```python
from build123d import *

# Parameters (mm, degrees)
F0_W     = 100
F0_H     = 100
F1_DEPTH = 100
F2_R     = 5
F3_DEPTH = 10
F4_R     = 5
F5_DEPTH = 10
F7_D     = 10


with BuildPart() as f1:
    # F0 (on Front) → F1 (new body)
    with BuildSketch(Plane.XZ):
        Rectangle(F0_W, F0_H)
    extrude(amount=F1_DEPTH)

    # F2 (on face) → F3 (join)
    with BuildSketch(Plane.XZ.offset(100)):
        Circle(F2_R)
    extrude(amount=F3_DEPTH)

    # F4 (on face) → F5 (join)
    with BuildSketch(Plane(origin=(0, 0, -50), x_dir=(1, 0, 0), z_dir=(0, 0, -1))):
        with Locations((0.200286, 29.510024)):
            Circle(F4_R)
    extrude(amount=F5_DEPTH)

    # F7 (through all)
    with Locations(Plane.YZ.offset(50)):
        with Locations((-50.594613, 0)):
            Hole(F7_D / 2)


solid = f1.part
```
Geometry check sheet. Reference: the model listing, model coordinates, mm. A direction names the side the tool comes from. Round coordinates to 2 decimals unless told otherwise and drop trailing zeros. Loops run counter-clockwise (first coordinate to the right, second up) from the corner with the lowest first, then second, coordinate; pieces in that order, holes last. Notation, with made-up numbers: (1.5, 13) -> (21.5, 13) arc R19 ccw to (21.5, 39) -> close; hole circle Ø1 at (-23.75, -3.75). An arc over 180 degrees is marked (long way). Use a Markdown table: item, result.
(1) Sectioned sample at D-D (x = 0). Enter the section's corners in (y, z), then the cut area to 3 significant figures.
Calculated:
| item | result |
|---|---|
| outline | (-110, -5) -> (-100, -5) -> (-100, -50) -> (-34.51, -50) -> (-34.51, -60) -> (-24.51, -60) -> (-24.51, -50) -> (0, -50) -> (0, 50) -> (-100, 50) -> (-100, 5) -> (-110, 5) -> close; hole circle Ø10 at (-50.59, 0) |
| area | 10,100 mm² |
(2) Sectioned sample at A-A (z = 0). Enter the section's corners in (x, y).
Calculated:
| item | result |
|---|---|
| outline | (-50, -100) -> (-5, -100) -> (-5, -110) -> (5, -110) -> (5, -100) -> (50, -100) -> (50, -55.59) -> (-50, -55.59) -> close; (-50, -45.59) -> (50, -45.59) -> (50, 0) -> (-50, 0) -> close |
(3) Scan lines: probe 1 along Z at (x, y) = (28.5, -59); probe 2 along Y at (x, z) = (10, -48.5). Record each from-to range of solid material in increasing order.
Calculated:
| item | result |
|---|---|
| probe 1 | -50 to 50 |
| probe 2 | -100 to 0 |
(4) Sectioned sample at C-C (y = -96). Enter the section's corners in (x, z), then the cut area to 3 significant figures.
Calculated:
| item | result |
|---|---|
| outline | (-50, -50) -> (50, -50) -> (50, 50) -> (-50, 50) -> close |
| area | 10,000 mm² |
(5) Go/stop test with flat-tipped pins: P1, Ø4, axis at x = 34.5, y = -97, coming from the -Z side; P2, Ø1.5, axis at x = 3, z = -11.5, coming from the -Y side; P3, Ø13, axis at y = -50.59, z = 0, coming from the +X side. Record where each tip stops, or that it passes through.
Calculated:
| item | result |
|---|---|
| P1 | z = -50 |
| P2 | y = -100 |
| P3 | x = 50 |
(6) Sectioned sample at B-B (x = -21.5). Enter the section's corners in (y, z), then the cut area to 3 significant figures.
Calculated:
| item | result |
|---|---|
| outline | (-100, -50) -> (0, -50) -> (0, 50) -> (-100, 50) -> close; hole circle Ø10 at (-50.59, 0) |
| area | 9,920 mm² |
(7) Mould release check, pull along Z, two halves, no side actions. Record for faces 1 (the cylindrical face through (-0.88, -24.63, -54.93)), 2 (the cylindrical face through (-0.7, -55.364, 1.502)), 3 (the flat face through (0, -30, -60)): released by +Z, released by -Z, zero draft, split by the parting line, or undercut.
Calculated:
| item | result |
|---|---|
| face 1 | zero draft |
| face 2 | undercut |
| face 3 | released by -Z |
(8) Set-up check for faces 4 (the cylindrical face through (-1.08, -104.93, -4.88)), 5 (the flat face through (50, -38, -1)): record each of +Z, -Z, +X, -X, +Y, -Y from which the full face is reachable in a straight line by a thin tool's end or side.
Calculated:
| item | result |
|---|---|
| face 4 | -Y |
| face 5 | +Z, -Z, +X, +Y, -Y |
